The listing builds one solid part. Answer for the finished solid, in the listing's coordinates (mm). A direction names the side the tool comes from. Round coordinates to 2 decimals unless told otherwise and drop trailing zeros. Write each loop counter-clockwise with the first axis right and the second up, starting at its lowest first coordinate (ties: lowest second). Pieces come first, ordered by that corner, then holes.
Item 1: For a pull along X with two mould halves and no side action, classify faces 1 (the face through (50, -1, 1)), 2 (the face through (41.5, -53, 0)), 3 (the face through (-45, 0, 4.25)) as +X half, -X half, draft (parallel to the pull), parting line (faces both ways), or undercut.
Item 2: Find the intervals of material crossed by probe 1 along Y at (x, z) = (15, -2); probe 2 along X at (y, z) = (35, 3.5); probe 3 along Z at (x, y) = (29, 47.95), in increasing order.
Item 3: Find section B-B on x = -5. Give the vertices of the cut face in (y, z).
Item 4: Find section A-A on y = 21.5. Give the vertices of the cut face in (x, z).
Item 5: A tool of negligible diameter and unlimited length cuts with its end or side. For faces 4 (the face through (-41.5, -53, 0)), 5 (the face through (46, 56.75, 0)), 6 (the face through (-41.5, 1, 0)), 7 (the face through (-50, -1, 1)), 8 (the face through (1, 50.25, 0)), from which of +Z, -Z, +X, -X, +Y, -Y can it reach the whole face along a straight path? Write none if from no direction.
Item 6: This flat-tipped pin is pushed along its axis until it touches: pin 1 (1.4 mm diameter, centred on x = -35.5, y = 47.75, fed in from -Z). Where does it stop, or does it pass through?
```python
from build123d import *

# Parameters (mm, degrees)
SKETCH1_W           = 100
SKETCH1_H           = 113.5
BOSS_EXTRUDE1_DEPTH = 4.25
CUT_EXTRUDE1_DEPTH  = 77.110528181
M2_HOLE1_C_D        = 1.6
M2_HOLE1_C_DEPTH    = 3
M2_HOLE1_C_TIP      = 0.480688495
M2_HOLE2_D_D        = 1.6
M2_HOLE2_D_DEPTH    = 5
M2_HOLE2_D_TIP      = 0.480688495
M2_HOLE3_E_D        = 1.6
M2_HOLE3_E_DEPTH    = 4
M2_HOLE3_E_TIP      = 0.480688495
M2_HOLE4_F_D        = 1.6
M2_HOLE4_F_DEPTH    = 10
M2_HOLE4_F_TIP      = 0.480688495
M2_HOLE5_G_D        = 1.6
M2_HOLE5_G_DEPTH    = 10
M2_HOLE5_G_TIP      = 0.480688495
M2_HOLE6_H_D        = 1.6
M2_HOLE6_H_DEPTH    = 5
M2_HOLE6_H_TIP      = 0.480688495
FILLET1_R           = 1
CHAMFER1_SIZE       = 1


with BuildPart() as part:
    # Sketch1 → Boss-Extrude1 (new, symmetric)
    with BuildSketch(Plane.XY):
        Rectangle(SKETCH1_W, SKETCH1_H)
    extrude(amount=BOSS_EXTRUDE1_DEPTH, both=True)

    # Sketch4 → Cut-Extrude1 (cut, through all)
    with BuildSketch(Plane.XY.offset(4.25)):
        with BuildLine():
            Line((-40.5, -44.75), (40.5, -44.75))
            ThreePointArc((40.5, -44.75), (41.207106781, -44.457106781), (41.5, -43.75))
            Line((41.5, -43.75), (41.5, 44.25))
            ThreePointArc((41.5, 44.25), (41.207106781, 44.957106781), (40.5, 45.25))
            Line((40.5, 45.25), (-40.5, 45.25))
            ThreePointArc((-40.5, 45.25), (-41.207106781, 44.957106781), (-41.5, 44.25))
            Line((-41.5, 44.25), (-41.5, -43.75))
            ThreePointArc((-41.5, -43.75), (-41.207106781, -44.457106781), (-40.5, -44.75))
        make_face()
        with BuildLine():
            Line((-41.5, 56.75), (41.5, 56.75))
            Line((41.5, 56.75), (41.5, 51.25))
            ThreePointArc((41.5, 51.25), (41.207106781, 50.542893219), (40.5, 50.25))
            Line((40.5, 50.25), (-40.5, 50.25))
            ThreePointArc((-40.5, 50.25), (-41.207106781, 50.542893219), (-41.5, 51.25))
            Line((-41.5, 51.25), (-41.5, 56.75))
        make_face()
        with BuildLine():
            Line((-41.5, -56.75), (41.5, -56.75))
            Line((41.5, -56.75), (41.5, -50.75))
            ThreePointArc((41.5, -50.75), (41.207106781, -50.042893219), (40.5, -49.75))
            Line((40.5, -49.75), (-40.5, -49.75))
            ThreePointArc((-40.5, -49.75), (-41.207106781, -50.042893219), (-41.5, -50.75))
            Line((-41.5, -50.75), (-41.5, -56.75))
        make_face()
    extrude(amount=-CUT_EXTRUDE1_DEPTH, mode=Mode.SUBTRACT)

    # M2 Hole1-C
    with Locations(Plane.XY.offset(4.25)):
        with Locations((-45.75, -40.75), (45.75, -40.75), (-45.75, 41.25), (45.75, 41.25)):
            Hole(M2_HOLE1_C_D / 2, depth=M2_HOLE1_C_DEPTH)
            with Locations((0, 0, -(M2_HOLE1_C_DEPTH + M2_HOLE1_C_TIP / 2))):  # 118° drill point
                Cone(0, M2_HOLE1_C_D / 2, M2_HOLE1_C_TIP, mode=Mode.SUBTRACT)

    # M2 Hole2-D
    with Locations(Plane.XY.offset(4.25)):
        with Locations((-21.5, 47.75), (21.5, 47.75), (-21.5, -47.25), (21.5, -47.25)):
            Hole(M2_HOLE2_D_D / 2, depth=M2_HOLE2_D_DEPTH)
            with Locations((0, 0, -(M2_HOLE2_D_DEPTH + M2_HOLE2_D_TIP / 2))):  # 118° drill point
                Cone(0, M2_HOLE2_D_D / 2, M2_HOLE2_D_TIP, mode=Mode.SUBTRACT)

    # M2 Hole3-E
    with Locations(Plane.XY.offset(4.25)):
        with Locations((0, 47.75), (0, -47.25)):
            Hole(M2_HOLE3_E_D / 2, depth=M2_HOLE3_E_DEPTH)
            with Locations((0, 0, -(M2_HOLE3_E_DEPTH + M2_HOLE3_E_TIP / 2))):  # 118° drill point
                Cone(0, M2_HOLE3_E_D / 2, M2_HOLE3_E_TIP, mode=Mode.SUBTRACT)

    # M2 Hole4-F
    with Locations(Plane(origin=(0, 50.25, 0), x_dir=(1, 0, 0), z_dir=(0, 1, 0))):
        with Locations((-29, 0), (29, 0)):
            Hole(M2_HOLE4_F_D / 2, depth=M2_HOLE4_F_DEPTH)
            with Locations((0, 0, -(M2_HOLE4_F_DEPTH + M2_HOLE4_F_TIP / 2))):  # 118° drill point
                Cone(0, M2_HOLE4_F_D / 2, M2_HOLE4_F_TIP, mode=Mode.SUBTRACT)

    # M2 Hole5-G
    with Locations(Plane(origin=(0, -49.75, 0), x_dir=(-1, 0, 0), z_dir=(0, -1, 0))):
        with Locations((29, 0), (-29, 0)):
            Hole(M2_HOLE5_G_D / 2, depth=M2_HOLE5_G_DEPTH)
            with Locations((0, 0, -(M2_HOLE5_G_DEPTH + M2_HOLE5_G_TIP / 2))):  # 118° drill point
                Cone(0, M2_HOLE5_G_D / 2, M2_HOLE5_G_TIP, mode=Mode.SUBTRACT)

    # M2 Hole6-H
    with Locations(Plane(origin=(0, 0, -4.25), x_dir=(-1, 0, 0), z_dir=(0, 0, -1))):
        with Locations((-35.5, 47.75), (35.5, 47.75), (-35.5, -47.25), (35.5, -47.25)):
            Hole(M2_HOLE6_H_D / 2, depth=M2_HOLE6_H_DEPTH)
            with Locations((0, 0, -(M2_HOLE6_H_DEPTH + M2_HOLE6_H_TIP / 2))):  # 118° drill point
                Cone(0, M2_HOLE6_H_D / 2, M2_HOLE6_H_TIP, mode=Mode.SUBTRACT)

    # Fillet1
    fillet1_edges = [part.edges().sort_by_distance(p)[0] for p in [
        (-50, 0, -4.25),
        (50, 0, -4.25),
    ]]
    fillet(fillet1_edges, radius=FILLET1_R)

    # Chamfer1
    chamfer1_edges = [part.edges().sort_by_distance(p)[0] for p in [
        (-45.75, -56.75, 4.25),
        (45.25, -56.75, -4.25),
        (45.75, -56.75, 4.25),
        (-45.25, -56.75, -4.25),
        (-49.707106781, -56.75, -3.957106781),
        (45.25, 56.75, -4.25),
        (-49.707106781, 56.75, -3.957106781),
        (49.707106781, 56.75, -3.957106781),
        (49.707106781, -56.75, -3.957106781),
        (41.5, -56.75, 0),
        (-41.5, -56.75, 0),
        (-45.25, 56.75, -4.25),
        (-45.75, 56.75, 4.25),
        (-41.5, 56.75, 0),
        (41.5, 56.75, 0),
        (45.75, 56.75, 4.25),
        (50, -56.75, 0.5),
        (-50, -56.75, 0.5),
        (-50, 56.75, 0.5),
        (50, 56.75, 0.5),
    ]]
    chamfer(chamfer1_edges, length=CHAMFER1_SIZE - 0.0001)  # a hair under: the kernel refuses the full size


solid = part.part
```
Check values:
1. face 1: +X half
1. face 2: undercut
1. face 3: draft
2. probe 1: y = -49.75 to -44.75, 45.25 to 50.25
2. probe 2: x = -50 to -41.5, 41.5 to 50
2. probe 3: z = -4.25 to -0.8, 0.8 to 4.25
3. outline: (-49.75, -4.25) - (-44.75, -4.25) - (-44.75, 4.25) - (-49.75, 4.25) - close; (45.25, -4.25) - (50.25, -4.25) - (50.25, 4.25) - (45.25, 4.25) - close
4. outline: (-50, -3.25) arc R1 ccw to (-49, -4.25) - (-41.5, -4.25) - (-41.5, 4.25) - (-50, 4.25) - close; (41.5, -4.25) - (49, -4.25) arc R1 ccw to (50, -3.25) - (50, 4.25) - (41.5, 4.25) - close
5. face 4: +Z, -Z, -Y
5. face 5: +Z, -Z, +X, -X, +Y
5. face 6: +Z, -Z
5. face 7: +Z, -Z, -X, +Y, -Y
5. face 8: +Z, -Z, +Y
6. pin 1: stops at z = 0.81
